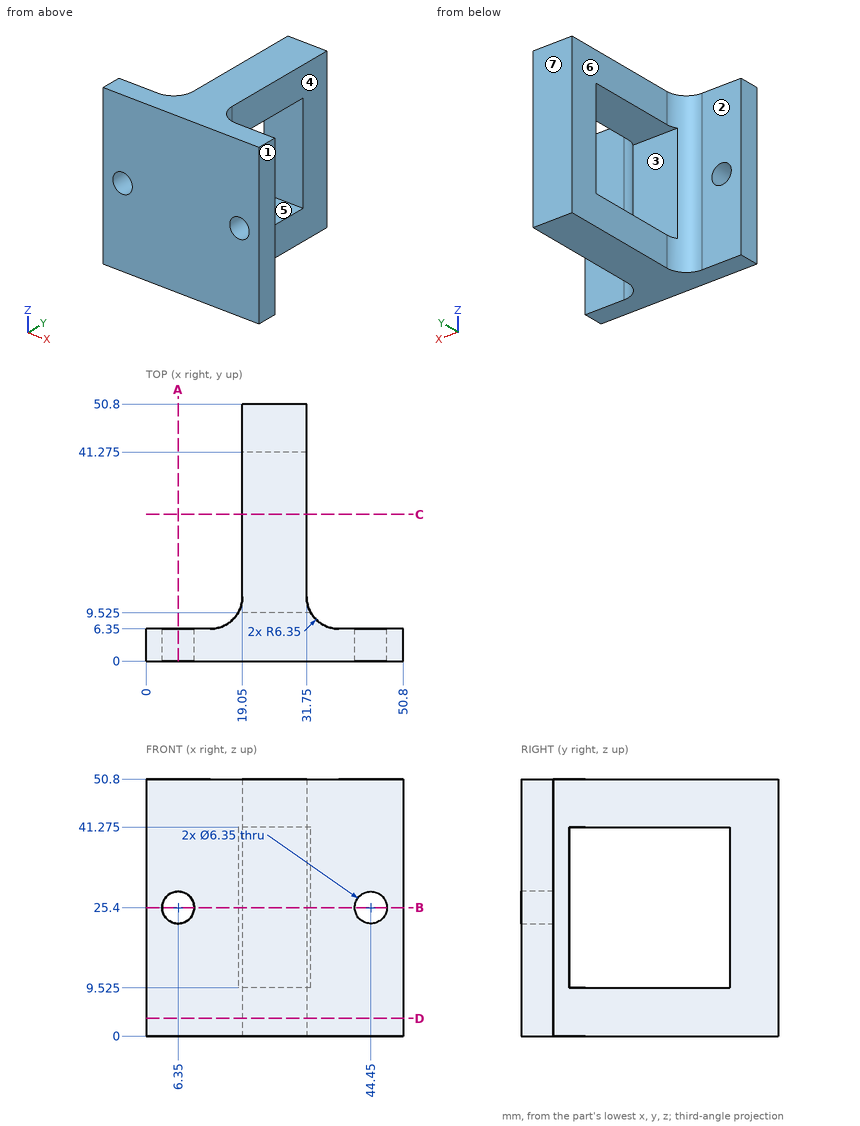
Print and shaded views of the part. All mm, measured from the part's lowest x, y and z. A direction names the side the tool comes from. Give positions to 0.01 mm unless a question says otherwise; leave off trailing zeros. Order: outer loops, then holes, each group sorted by start corner. A loop starts at its lowest first (then second) coordinate and runs counter-clockwise, first axis right, second up. Notation, with made-up numbers: (66.25, 7) -> (95.25, 7) arc R29 cw to (95.25, 37) -> close; hole circle Ø5 at (-20.5, -5). An arc over 180 degrees is marked (long way). Use CSV: the item, a comma, the result in double quotes.
1. Band-saw the part on C-C, the plane y = 29. Give the cut face in (x, z) (3 decimals), then the cut area to 3 significant figures.
Outcome:
outline,"(19.05, 0) -> (31.75, 0) -> (31.75, 9.525) -> (19.05, 9.525) -> close; (19.05, 41.275) -> (31.75, 41.275) -> (31.75, 50.8) -> (19.05, 50.8) -> close"
area,"242 mm²"
2. Mould opens along Y. For the marked faces 5, 6 and 7 say: +Y half, -Y half, draft (parallel to the pull), parting line (faces both ways), or undercut.
Outcome:
face 5,"undercut"
face 6,"draft"
face 7,"+Y half"
3. Band-saw the part on A-A, the plane x = 6.35. Give the cut face in (y, z) (3 decimals), then the cut area to 3 significant figures.
Outcome:
outline,"(0, 0) -> (6.35, 0) -> (6.35, 22.225) -> (0, 22.225) -> close; (0, 28.575) -> (6.35, 28.575) -> (6.35, 50.8) -> (0, 50.8) -> close"
area,"282 mm²"
4. Drop flat-ended pins along their axis: pin 1 (1.5 mm diameter, centred on y = 26, z = 42, fed in from +X); pin 2 (1 mm diameter, centred on x = 16.5, z = 36, fed in from +Y); pin 3 (14 mm diameter, centred on x = 3, z = 30, fed in from +Y). Give the stop position or say it passes through.
Outcome:
pin 1,"x = 31.75"
pin 2,"y = 8.03"
pin 3,"y = 6.35"
5. Band-saw the part on D-D, the plane z = 3.5. Give the cut face in (x, y), then the cut area to 3 significant figures.
Outcome:
outline,"(0, 0) -> (50.8, 0) -> (50.8, 6.35) -> (38.1, 6.35) arc R6.35 cw to (31.75, 12.7) -> (31.75, 50.8) -> (19.05, 50.8) -> (19.05, 12.7) arc R6.35 cw to (12.7, 6.35) -> (0, 6.35) -> close"
area,"904 mm²"
6. Band-saw the part on B-B, the plane z = 25.4. Give the cut face in (x, y) (3 decimals), then the cut area to 3 significant figures.
Outcome:
outline,"(0, 0) -> (3.175, 0) -> (3.175, 6.35) -> (0, 6.35) -> close; (9.525, 0) -> (41.275, 0) -> (41.275, 6.35) -> (38.1, 6.35) arc R6.35 cw to (32.601, 9.525) -> (18.199, 9.525) arc R6.35 cw to (12.7, 6.35) -> (9.525, 6.35) -> close; (19.05, 41.275) -> (31.75, 41.275) -> (31.75, 50.8) -> (19.05, 50.8) -> close; (47.625, 0) -> (50.8, 0) -> (50.8, 6.35) -> (47.625, 6.35) -> close"
area,"419 mm²"
7. Drill centre lines: line 1 along X through (y, z) = (3.75, 25.4) (3 decimals); line 2 along Z through (x, y) = (20, 23.5) (3 decimals). Where is each one in solid material? Low to high. Write a range as from..to.
Outcome:
line 1,"0..3.175, 9.525..41.275, 47.625..50.8"
line 2,"0..9.525, 41.275..50.8"
8. 3-axis set-ups, long thin cutter, end or side, ignore diameter. For the marked faces 1, 2, 3 and 4: which of +Z, -Z, +X, -X, +Y, -Y reach the whole face in a straight line?
Outcome:
face 1,"+Z, -Z, +X, +Y, -Y"
face 2,"+Z, -Z, -X, +Y"
face 3,"+X, -X"
face 4,"+Z, -Z, +X, +Y"
